Geometry check sheet. Reference: the model listing, model coordinates, mm. A direction names the side the tool comes from. Round coordinates to 2 decimals unless told otherwise and drop trailing zeros. Order: outer loops, then holes, each group sorted by start corner. A loop starts at its lowest first (then second) coordinate and runs counter-clockwise, first axis right, second up. Notation, with made-up numbers: (22, 63.25) - (75, 63.25) arc R11 cw to (75, 77.25) - close; hole circle Ø5 at (18.5, 83). An arc over 180 degrees is marked (long way). Use a Markdown table: item, result. Add a question column.
(1) Section check D-D on z = 44. Record the boundary of the cut face in (x, y), then the cut area to 3 significant figures.
(2) Thickness scan on line 1 along X through (y, z) = (15.25, 0); line 2 along Y through (x, z) = (-35, -26). Record the ranges inside material, lowest first. Write a range as [from, to].
(3) Mould release check, pull along X, two halves, no side actions. Record for faces 1 (the face through (-39.033, 52.55, 4.107)), 2 (the face through (6.69, 39.95, -12.66)), 3 (the face through (11.42, 70.71, -31.91)), 4 (the face through (-33.34, 70.71, 6.07)): released by +X, released by -X, zero draft, split by the parting line, or undercut.
(4) Section check B-B on y = 9. Record the boundary of the cut face in (x, z) (1 decimal), then the cut area to 3 significant figures.
(5) Section check A-A on x = 1. Give the number of separate pieces and of enclosed holes in the cut face, then the cut area to 3 significant figures.
(6) Access from +Z, -Z, +X, -X, +Y, -Y to the whole of each face (thin tool, end or side, straight path). Record for faces 5 (the face through (-5.494, 60.17, -40.822)), 6 (the face through (-32.606, 60.17, 25.169)), 7 (the face through (23, 53, 0)), 8 (the face through (23, 53, 31.75)), 9 (the face through (-24.88, 78.53, 11.79)).
(7) Gauge pin test, flat ends, axial feed: P1, Ø8, axis at x = 9.5, z = -5.5, coming from the +Y side; P2, Ø5, axis at x = 6.5, y = 50, coming from the -Z side; P3, Ø2, axis at x = 22.86, y = 69.85, coming from the -Z side (3 decimals); P4, Ø3, axis at x = -5.5, y = 56.5, coming from the +Z side. Record the tip position at first contact, or that the pin passes through.
```python
from build123d import *

# Parameters (mm, degrees)
SKETCH1_R           = 50.8
BOSS_EXTRUDE1_DEPTH = 25.4
BOSS_EXTRUDE2_DEPTH = 31.75
SKETCH9_R           = 6.604
CUT_EXTRUDE2_DEPTH  = 68.58
SKETCH10_R          = 1.27
CUT_EXTRUDE3_DEPTH  = 68.58
CIRPATTERN3_COUNT   = 3
SKETCH11_R          = 4.7625
CUT_EXTRUDE4_DEPTH  = 25.4


with BuildPart() as part:
    # Sketch1 → Boss-Extrude1 (new body)
    with BuildSketch(Plane(origin=(0, 0, 0), x_dir=(1, 0, 0), z_dir=(0, 1, 0))):
        Circle(SKETCH1_R)
    extrude(amount=BOSS_EXTRUDE1_DEPTH)

    # Sketch4 → Boss-Extrude2 (add)
    with BuildSketch(Plane.XY):
        Polygon((7.62, 25.4), (7.62, 63.5), (38.1, 93.98), (38.1, 25.4), align=None)
    boss_extrude2 = extrude(amount=BOSS_EXTRUDE2_DEPTH)

    # Sketch9 → Cut-Extrude2 (cut)
    with BuildSketch(Plane(origin=(66.802, 66.802, 0), x_dir=(0, 0, -1), z_dir=(0.707106781, 0.707106781, 0))):
        with Locations((-15.875, 29.160757667)):
            Circle(SKETCH9_R)
    cut_extrude2 = extrude(amount=-CUT_EXTRUDE2_DEPTH, mode=Mode.SUBTRACT)

    # Sketch10 → Cut-Extrude3 (cut)
    with BuildSketch(Plane.XY.offset(31.75)):
        with Locations((22.86, 69.85)):
            Circle(SKETCH10_R)
    cut_extrude3 = extrude(amount=-CUT_EXTRUDE3_DEPTH, mode=Mode.SUBTRACT)

    # CirPattern3: Boss-Extrude2, Cut-Extrude2, Cut-Extrude3 ×3 about axis
    cirpattern3_axis = Axis((0, 0, 0), (0, 1, 0))
    for i in range(1, CIRPATTERN3_COUNT):
        add(boss_extrude2.rotate(cirpattern3_axis, i * 360 / CIRPATTERN3_COUNT))
        add(cut_extrude2.rotate(cirpattern3_axis, i * 360 / CIRPATTERN3_COUNT), mode=Mode.SUBTRACT)
        add(cut_extrude3.rotate(cirpattern3_axis, i * 360 / CIRPATTERN3_COUNT), mode=Mode.SUBTRACT)

    # Sketch11 → Cut-Extrude4 (cut)
    with BuildSketch(Plane(origin=(0, 25.4, 0), x_dir=(1, 0, 0), z_dir=(0, 1, 0))):
        Circle(SKETCH11_R)
    extrude(amount=-CUT_EXTRUDE4_DEPTH, mode=Mode.SUBTRACT)


solid = part.part
```
Check sheet entries:
| question | item | result |
|---|---|---|
| 1 | outline | (-25.39, 0) - (25.39, 0) - (25.39, 25.4) - (-25.39, 25.4) - close |
| 1 | area | 1,290 mm2 |
| 2 | line 1 | x = [-50.8, -4.76], [4.76, 50.8] |
| 2 | line 2 | y = [0, 25.4] |
| 3 | face 1 | released by -X |
| 3 | face 2 | released by +X |
| 3 | face 3 | undercut |
| 3 | face 4 | undercut |
| 4 | outline | circle Ø101.6 at (0, 0); hole circle Ø9.5 at (0, 0) |
| 4 | area | 8,040 mm2 |
| 5 | separate pieces | 2 |
| 5 | enclosed holes | 1 |
| 5 | area | 3,830 mm2 |
| 6 | face 5 | -Z, -X, +Y |
| 6 | face 6 | +Z, -X, +Y |
| 6 | face 7 | +X, +Y |
| 6 | face 8 | +Z, +X, +Y |
| 6 | face 9 | +Y |
| 7 | P1 | stops at y = 25.4 |
| 7 | P2 | stops at z = -48.87 |
| 7 | P3 | passes through |
| 7 | P4 | stops at z = 12.12 |
